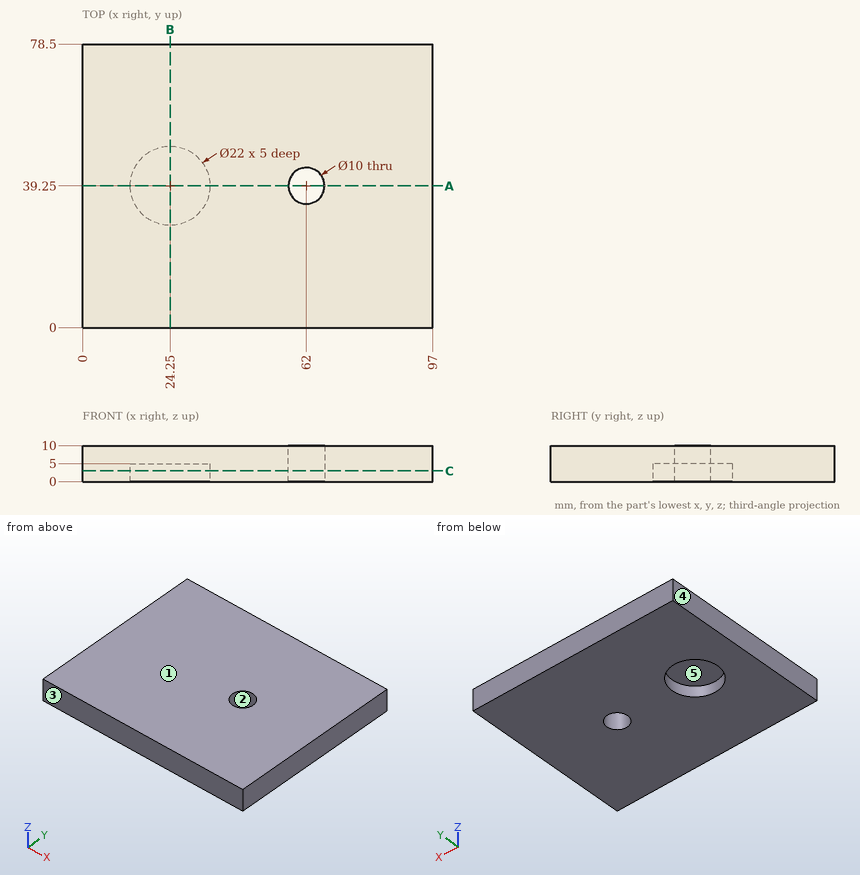
Input: dimensioned drawing with shaded views. Units: mm. Origin: part minimum x, y, z. A direction names the side the tool comes from. Coordinates: 2 decimals unless noted, no trailing zeros. Order: outer loops, then holes, each group sorted by start corner. A loop starts at its lowest first (then second) coordinate and runs counter-clockwise, first axis right, second up. Notation, with made-up numbers: (43.25, -4.5) -> (48.25, -4.5) arc R22 ccw to (48.25, 31.5) -> close; hole circle Ø6 at (10, -7). An arc over 180 degrees is marked (long way). Answer in a Markdown table with one row per item.
Item 1: Section B-B on x = 24.25. Output: boundary loops of the cut face in (y, z).
Return value:
| item | result |
|---|---|
| outline | (0, 0) -> (28.25, 0) -> (28.25, 5) -> (50.25, 5) -> (50.25, 0) -> (78.5, 0) -> (78.5, 10) -> (0, 10) -> close |
Item 2: Ray query, L1, parallel to Y at x = 62, z = 2.5; L2, parallel to Z at x = 32, y = 38.5; L3, parallel to Y at x = 30, z = 4. Return the intervals inside material, ascending.
Return value:
| item | result |
|---|---|
| L1 | y = 0 to 34.25, 44.25 to 78.5 |
| L2 | z = 5 to 10 |
| L3 | y = 0 to 29.87, 48.63 to 78.5 |
Item 3: Section C-C on z = 3. Output: boundary loops of the cut face in (x, y).
Return value:
| item | result |
|---|---|
| outline | (0, 0) -> (97, 0) -> (97, 78.5) -> (0, 78.5) -> close; hole circle Ø22 at (24.25, 39.25); hole circle Ø10 at (62, 39.25) |
Item 4: Contact query for a flat-ended pin moving along its axis: P1, Ø24, axis at x = 28.5, y = 37.5, coming from the -Z side. Output: stop coordinate, or through.
Return value:
| item | result |
|---|---|
| P1 | stops at z = 0 |
Item 5: Section A-A on y = 39.25. Output: boundary loops of the cut face in (x, z), plus the area to 3 significant figures.
Return value:
| item | result |
|---|---|
| outline | (0, 0) -> (13.25, 0) -> (13.25, 5) -> (35.25, 5) -> (35.25, 0) -> (57, 0) -> (57, 10) -> (0, 10) -> close; (67, 0) -> (97, 0) -> (97, 10) -> (67, 10) -> close |
| area | 760 mm² |
Item 6: Draft query along Y for the marked faces 1, 2 and 3. Return one class per face: released by +Y, released by -Y, zero draft, split by the parting line, or undercut.
Return value:
| item | result |
|---|---|
| face 1 | zero draft |
| face 2 | undercut |
| face 3 | released by -Y |
Item 7: Access query for the marked faces 4 and 5. Directions: +Z, -Z, +X, -X, +Y, -Y. A direction counts if a zero-diameter tool reaches every point of the face in a straight line with its end or side. Return the directions, or none.
Return value:
| item | result |
|---|---|
| face 4 | +Z, -Z, -X, +Y, -Y |
| face 5 | -Z |
